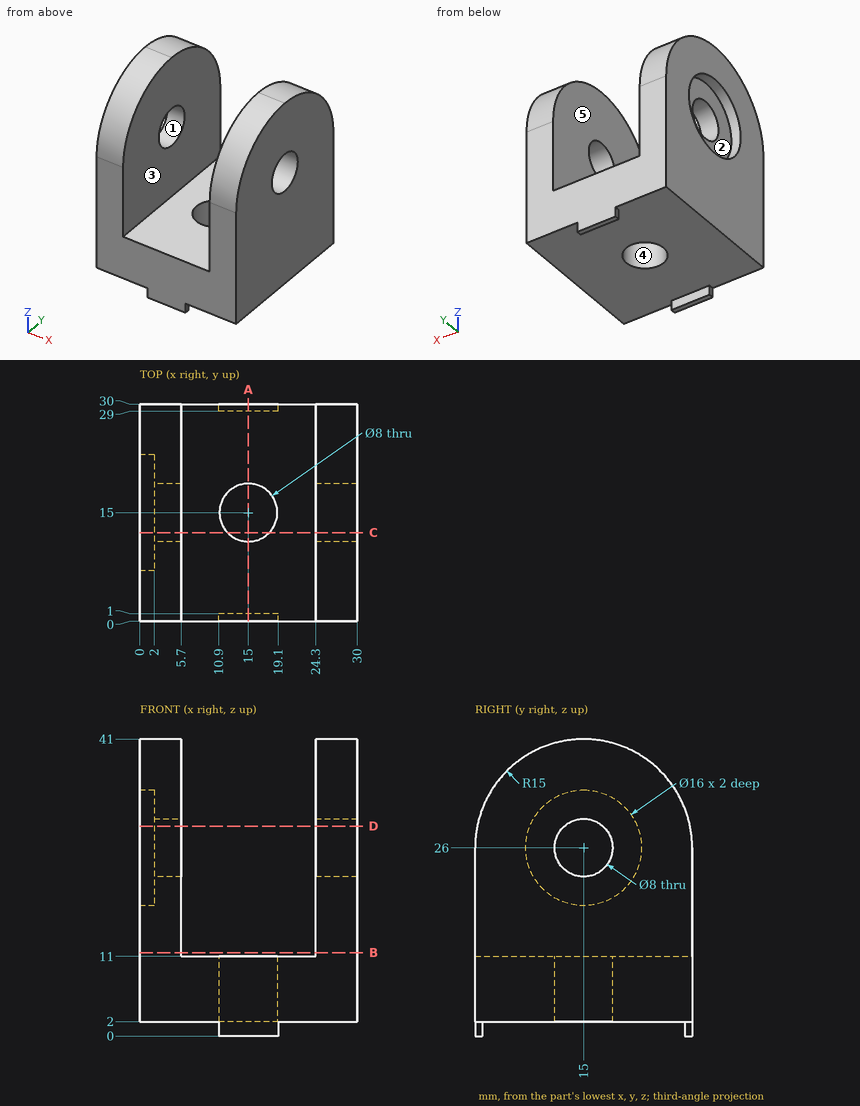
Verification items for this drawing (mm, ordinates from the low corner). A direction names the side the tool comes from. Give positions to 0.01 mm unless a question says otherwise; leave off trailing zeros. Order: outer loops, then holes, each group sorted by start corner. A loop starts at its lowest first (then second) coordinate and runs counter-clockwise, first axis right, second up.
1) Tool access check on the marked faces 4 and 5. Record the directions out of +Z, -Z, +X, -X, +Y, -Y that give a thin tool (end or side, any length) a straight path to the whole face; none if there is none.
Results are:
face 4: +Z, -Z
face 5: +Z, +Y, -Y
2) Material ranges on probe 1 along X at (y, z) = (18.75, 23.5); probe 2 along X at (y, z) = (14, 14); probe 3 along Y at (x, z) = (0.65, 26), recorded low to high.
Results are:
probe 1: x = 2 to 5.7, 24.3 to 30
probe 2: x = 0 to 5.7, 24.3 to 30
probe 3: y = 0 to 7, 23 to 30
3) Cross-section at C-C (y = 12.25). Record the boundary of the cut face in (x, z).
Results are:
outline: (0, 2) - (12.1, 2) - (12.1, 11) - (5.7, 11) - (5.7, 23.1) - (2, 23.1) - (2, 18.49) - (0, 18.49) - close; (0, 33.51) - (2, 33.51) - (2, 28.9) - (5.7, 28.9) - (5.7, 40.75) - (0, 40.75) - close; (17.9, 2) - (30, 2) - (30, 23.1) - (24.3, 23.1) - (24.3, 11) - (17.9, 11) - close; (24.3, 28.9) - (30, 28.9) - (30, 40.75) - (24.3, 40.75) - close
4) Cross-section at A-A (x = 15). Record the boundary of the cut face in (y, z).
Results are:
outline: (0, 0) - (1, 0) - (1, 2) - (11, 2) - (11, 11) - (0, 11) - close; (19, 2) - (29, 2) - (29, 0) - (30, 0) - (30, 11) - (19, 11) - close
5) Gauge pin test, flat ends, axial feed: pin 1 (1.5 mm diameter, centred on x = 11, y = 12, fed in from +Z); pin 2 (1.1 mm diameter, centred on y = 0.5, z = 0.5, fed in from +X); pin 3 (15 mm diameter, centred on x = 19, y = 21, fed in from +Z); pin 4 (7 mm diameter, centred on y = 15, z = 26, fed in from -X). Record the tip position at first contact, or that the pin passes through.
Results are:
pin 1: stops at z = 11
pin 2: stops at x = 19.1
pin 3: stops at z = 40.98
pin 4: passes through
6) Cross-section at D-D (z = 29). Record the boundary of the cut face in (x, y).
Results are:
outline: (0, 0.3) - (5.7, 0.3) - (5.7, 12.35) - (2, 12.35) - (2, 7.58) - (0, 7.58) - close; (0, 22.42) - (2, 22.42) - (2, 17.65) - (5.7, 17.65) - (5.7, 29.7) - (0, 29.7) - close; (24.3, 0.3) - (30, 0.3) - (30, 12.35) - (24.3, 12.35) - close; (24.3, 17.65) - (30, 17.65) - (30, 29.7) - (24.3, 29.7) - close
7) Draft check along X on the marked faces 1, 2 and 3. Enter one of: released by +X, released by -X, zero draft, split by the parting line, or undercut.
Results are:
face 1: zero draft
face 2: released by -X
face 3: undercut
8) Cross-section at B-B (z = 11.5). Record the boundary of the cut face in (x, y).
Results are:
outline: (0, 0) - (5.7, 0) - (5.7, 30) - (0, 30) - close; (24.3, 0) - (30, 0) - (30, 30) - (24.3, 30) - close
